Geometry: final body of the model. Coordinates: model frame, mm. A direction names the side the tool comes from. Give positions to 0.01 mm unless a question says otherwise; leave off trailing zeros. Write each loop counter-clockwise with the first axis right and the second up, starting at its lowest first coordinate (ties: lowest second). Pieces come first, ordered by that corner, then holes.
from build123d import *

# Parameters (mm, degrees)
SKETCH1_R           = 6.5
BOSS_EXTRUDE1_DEPTH = 2.5
BOSS_EXTRUDE2_START = 2.5
SKETCH2_R           = 5
BOSS_EXTRUDE2_DEPTH = 2.5
FILLET1_R           = 10
FILLET2_R           = 1
CHAMFER1_SIZE       = 0.5
SKETCH3_R           = 2.85
CUT_EXTRUDE1_DEPTH  = 26.597851472
SKETCH4_R           = 1.6
CUT_EXTRUDE2_DEPTH  = 26.597851541


with BuildPart() as part:
    # Sketch1 → Boss-Extrude1 (new, symmetric)
    with BuildSketch(Plane(origin=(0, 0, 0), x_dir=(0, 0, -1), z_dir=(1, 0, 0))):
        with BuildLine():
            Line((-9.486832981, -6.5), (-17.5, -6.5))
            Line((-17.5, -6.5), (-17.5, -17.2))
            Line((-17.5, -17.2), (17.5, -17.2))
            Line((17.5, -17.2), (17.5, -6.5))
            Line((17.5, -6.5), (9.486832981, -6.5))
            ThreePointArc((9.486832981, -6.5), (0, 11.5), (-9.486832981, -6.5))
        make_face()
        Circle(SKETCH1_R, mode=Mode.SUBTRACT)
    extrude(amount=BOSS_EXTRUDE1_DEPTH, both=True)

    # Sketch2 → Boss-Extrude2 (add)
    with BuildSketch(Plane(origin=(2.5, 0, 0), x_dir=(0, 0, -1), z_dir=(1, 0, 0)).offset(BOSS_EXTRUDE2_START)):
        with BuildLine():
            Line((-9.486832981, -6.5), (-17.5, -6.5))
            Line((-17.5, -6.5), (-17.5, -17.2))
            Line((-17.5, -17.2), (17.5, -17.2))
            Line((17.5, -17.2), (17.5, -6.5))
            Line((17.5, -6.5), (9.486832981, -6.5))
            ThreePointArc((9.486832981, -6.5), (0, 11.5), (-9.486832981, -6.5))
        make_face()
        Circle(SKETCH2_R, mode=Mode.SUBTRACT)
    extrude(amount=-BOSS_EXTRUDE2_DEPTH)

    # Fillet1
    # the kernel refuses this fillet: 10 mm, written as the material it adds along each edge
    with BuildSketch(Plane(origin=(5, -6.5, 9.486832981), x_dir=(0, 0, 1), z_dir=(-1, 0, 0))) as fillet1_piece_1:
        with BuildLine():
            CenterArc((11.837899914, 9.239665486), FILLET1_R, 187.320893322, 60.192138393)
            Line((1.919419498, 7.965402469), (1.72104989, 7.939917209))
            ThreePointArc((1.72104989, 7.939917209), (1.498721871, 3.852815723), (-0.1649884, 0.113043478))
            Line((-0.1649884, 0.113043478), (0, -0.2))
            ThreePointArc((0, -0.2), (4.00658351, -0.2), (7.936672362, -0.18479331))
            Line((7.936672362, -0.18479331), (8.013167019, 0))
        make_face()
    extrude(amount=7.5)
    with BuildSketch(Plane(origin=(5, -6.5, -9.486832981), x_dir=(0, 0.9721729957330114, -0.23426409534434056), z_dir=(-1, 0, 0))) as fillet1_piece_2:
        with BuildLine():
            CenterArc((11.755748189, 9.343964746), FILLET1_R, 188.938720591, 60.192138393)
            Line((1.877197323, 7.790184587), (1.679626305, 7.759108983))
            ThreePointArc((1.679626305, 7.759108983), (0.744164062, 3.941945112), (-0.194434599, 0.046852819))
            Line((-0.194434599, 0.046852819), (0.071246959, -0.186879295))
            ThreePointArc((0.071246959, -0.186879295), (4.096700126, 0.554440542), (8.122153294, -0.186879295))
            Line((8.122153294, -0.186879295), (8.193400253, 0))
        make_face()
    extrude(amount=7.5)

    # Fillet2
    fillet2_edges = [part.edges().sort_by_distance(p)[0] for p in [
        (1.25, -6.5, -17.5),
        (1.25, -17.2, -17.5),
        (1.25, -17.2, 17.5),
        (1.25, -6.5, 17.5),
    ]]
    fillet(fillet2_edges, radius=FILLET2_R)

    # Chamfer1
    chamfer1_edges = [part.edges().sort_by_distance(p)[0] for p in [
        (-2.5, 0, 6.5),
        (5, 0, 5),
        (-2.5, 11.5, 0),
        (5, 11.5, 0),
        (-2.5, -3.089050017, -13.199089807),
        (5, -3.089050017, 13.199089807),
        (-2.5, -11.672887978, -17.5),
        (5, -11.672887978, -17.5),
        (-2.5, -17.2, 0),
        (-2.5, -11.672887978, 17.5),
        (-2.5, -3.089050017, 13.199089807),
        (-2.5, -6.61597037, 17.348119119),
        (-2.5, -16.907106781, 17.207106781),
        (-2.5, -6.61597037, -17.348119119),
        (-2.5, -16.907106781, -17.207106781),
        (5, -17.2, 0),
        (5, -3.089050017, -13.199089807),
        (5, -11.672887978, 17.5),
        (5, -6.61597037, 17.348119119),
        (5, -16.907106781, 17.207106781),
        (5, -6.61597037, -17.348119119),
        (5, -16.907106781, -17.207106781),
    ]]
    chamfer(chamfer1_edges, length=CHAMFER1_SIZE)

    # Sketch3 → Cut-Extrude1 (cut, through all)
    with BuildSketch(Plane(origin=(0, -6.5, 0), x_dir=(1, 0, 0), z_dir=(0, 1, 0))):
        with Locations((1.25, -14.5)):
            Circle(SKETCH3_R)
    cut_extrude1 = extrude(amount=CUT_EXTRUDE1_DEPTH, mode=Mode.SUBTRACT)

    # Sketch4 → Cut-Extrude2 (cut, through all)
    with BuildSketch(Plane(origin=(0, -6.5, 0), x_dir=(1, 0, 0), z_dir=(0, 1, 0))):
        with Locations(Location((1.25, -14.5, 0), (0, 0, 270))):
            Circle(SKETCH4_R)
    cut_extrude2 = extrude(amount=-CUT_EXTRUDE2_DEPTH, mode=Mode.SUBTRACT)

    # Mirror1: Cut-Extrude1, Cut-Extrude2 across plane
    add(cut_extrude1.mirror(Plane.XY), mode=Mode.SUBTRACT)
    add(cut_extrude2.mirror(Plane.XY), mode=Mode.SUBTRACT)


solid = part.part
Q1. Section A-A on x = 1.25. Output: boundary loops of the cut face in (y, z).
Filled sheet:
outline: (-17.2, -16.5) arc R1 ccw to (-16.2, -17.5) - (-7.15, -17.5) arc R1 ccw to (-6.5, -17.26) - (-6.5, -16.1) - (-17.2, -16.1) - close; (-17.2, -12.9) - (-6.5, -12.9) - (-6.5, -11.65) - (0.21, -11.65) arc R10 cw to (1.47, -11.41) arc R11.5 ccw to (1.47, 11.41) arc R10 cw to (0.21, 11.65) - (-6.5, 11.65) - (-6.5, 12.9) - (-17.2, 12.9) - close; (-17.2, 16.1) - (-6.5, 16.1) - (-6.5, 17.26) arc R1 ccw to (-7.15, 17.5) - (-16.2, 17.5) arc R1 ccw to (-17.2, 16.5) - close; hole circle Ø13 at (0, 0)
Q2. Pull-direction query (Z, two-part tool) for faces 4 (the cylindrical face through (1.296, -6.718, 17.404)), 5 (the flat face through (0, -6.5, -16)), 6 (the conical face through (-2.309, -16.694, -16.983)); classes: released by +Z, released by -Z, zero draft, split by the parting line, or undercut.
Filled sheet:
face 4: released by +Z
face 5: undercut
face 6: released by -Z
Q3. Pin query (flat end, axial travel): P1, Ø10.5, axis at y = 0, z = 0, coming from the -X side; P2, Ø3.5, axis at x = 1.25, z = -14.5, coming from the -Y side; P3, Ø1, axis at x = -0.5, z = 7, coming from the +Y side. Return the tip coordinate at first contact, or that it passes through.
Filled sheet:
P1: stops at x = 2.5
P2: stops at y = -17.2
P3: stops at y = 9.49
Q4. Section C-C on z = 0. Output: boundary loops of the cut face in (x, y).
Filled sheet:
outline: (-2.5, -16.7) - (-2, -17.2) - (4.5, -17.2) - (5, -16.7) - (5, -5.5) - (4.5, -5) - (2.5, -5) - (2.5, -6.5) - (-2, -6.5) - (-2.5, -7) - close; (-2.5, 7) - (-2, 6.5) - (2.5, 6.5) - (2.5, 5) - (4.5, 5) - (5, 5.5) - (5, 11) - (4.5, 11.5) - (-2, 11.5) - (-2.5, 11) - close
Q5. Section D-D on x = 3.5. Output: boundary loops of the cut face in (y, z), plus the area to 3 significant figures.
Filled sheet:
outline: (-17.2, -16.5) arc R1 ccw to (-16.2, -17.5) - (-7.15, -17.5) arc R1 ccw to (-6.25, -16.94) arc R10 cw to (-5.88, -16.25) - (-6.5, -16.25) - (-6.5, -12.75) - (-2.41, -12.75) arc R10 cw to (1.47, -11.41) arc R11.5 ccw to (1.47, 11.41) arc R10 cw to (-2.41, 12.75) - (-6.5, 12.75) - (-6.5, 16.25) - (-5.88, 16.25) arc R10 cw to (-6.25, 16.94) arc R1 ccw to (-7.15, 17.5) - (-16.2, 17.5) arc R1 ccw to (-17.2, 16.5) - close; hole circle Ø10 at (0, 0)
area: 667 mm2
Q6. Access query for faces 1 (the flat face through (1, -12, 17.5)), 2 (the flat face through (2.5, -5, -2)), 3 (the flat face through (0, -6.5, 16)). Directions: +Z, -Z, +X, -X, +Y, -Y. A direction counts if a zero-diameter tool reaches every point of the face in a straight line with its end or side. Return the directions, or none.
Filled sheet:
face 1: +Z, +X, -X, +Y, -Y
face 2: -X
face 3: +Y
Q7. Section B-B on y = -9.5. Output: boundary loops of the cut face in (x, z).
Filled sheet:
outline: (-2.5, -17) - (-2, -17.5) - (4.5, -17.5) - (5, -17) - (5, 17) - (4.5, 17.5) - (-2, 17.5) - (-2.5, 17) - close; hole circle Ø3.2 at (1.25, -14.5); hole circle Ø3.2 at (1.25, 14.5)
Q8. Ray query, line 1 along Y through (x, z) = (1.15, 0); line 2 along X through (y, z) = (-14, -14.5); line 3 along Y through (x, z) = (3.2, 0). Return the intervals inside material, ascending.
Filled sheet:
line 1: y = -17.2 to -6.5, 6.5 to 11.5
line 2: x = -2.5 to -0.35, 2.85 to 5
line 3: y = -17.2 to -5, 5 to 11.5
